```python
from build123d import *

# Parameters (mm, degrees)
BOSS_EXTRUDE1_DEPTH = 50.8
SKETCH2_R           = 8.636
SKETCH2_R_2         = 4.064
CUT_EXTRUDE1_DEPTH  = 50.8
CIRPATTERN1_COUNT   = 4


with BuildPart() as part:
    # Sketch1 → Boss-Extrude1 (new body)
    with BuildSketch(Plane.XY):
        with BuildLine():
            Line((-3.797752579, 127.26397791), (-3.797752579, 92.878939343))
            ThreePointArc((-3.797752579, 92.878939343), (0, 89.081186764), (3.797752579, 92.878939343))
            Line((3.797752579, 92.878939343), (3.797752579, 127.26397791))
            ThreePointArc((3.797752579, 127.26397791), (6.790630722, 127.103835386), (9.749331178, 126.62523659))
            ThreePointArc((9.749331178, 126.62523659), (30.88440355, 95.052420362), (66.541072029, 108.172481405))
            ThreePointArc((66.541072029, 108.172481405), (69.216024294, 106.82059547), (71.731442986, 105.190983859))
            Line((71.731442986, 105.190983859), (51.520424417, 77.372903306))
            ThreePointArc((51.520424417, 77.372903306), (52.360607836, 72.068193971), (57.665317172, 72.90837739))
            Line((57.665317172, 72.90837739), (77.876335741, 100.726457943))
            ThreePointArc((77.876335741, 100.726457943), (80.203495606, 98.837730286), (82.315821243, 96.711455232))
            ThreePointArc((82.315821243, 96.711455232), (80.856418217, 58.745626497), (117.415047369, 48.40151497))
            ThreePointArc((117.415047369, 48.40151497), (118.784510595, 45.735518782), (119.861665394, 42.938609284))
            Line((119.861665394, 42.938609284), (87.159550401, 32.313048015))
            ThreePointArc((87.159550401, 32.313048015), (84.721243151, 27.527600589), (89.506690576, 25.089293339))
            Line((89.506690576, 25.089293339), (122.208805569, 35.714854608))
            ThreePointArc((122.208805569, 35.714854608), (122.981351186, 32.818971587), (123.440465405, 29.857185076))
            ThreePointArc((123.440465405, 29.857185076), (99.944029333, 0), (123.440465405, -29.857185076))
            ThreePointArc((123.440465405, -29.857185076), (122.981351186, -32.818971587), (122.208805569, -35.714854608))
            Line((122.208805569, -35.714854608), (89.506690576, -25.089293339))
            ThreePointArc((89.506690576, -25.089293339), (84.721243151, -27.527600589), (87.159550401, -32.313048015))
            Line((87.159550401, -32.313048015), (119.861665394, -42.938609284))
            ThreePointArc((119.861665394, -42.938609284), (118.784510595, -45.735518782), (117.415047369, -48.40151497))
            ThreePointArc((117.415047369, -48.40151497), (80.856418217, -58.745626497), (82.315821243, -96.711455232))
            ThreePointArc((82.315821243, -96.711455232), (80.203495606, -98.837730286), (77.876335741, -100.726457943))
            Line((77.876335741, -100.726457943), (57.665317172, -72.90837739))
            ThreePointArc((57.665317172, -72.90837739), (52.360607836, -72.068193971), (51.520424417, -77.372903306))
            Line((51.520424417, -77.372903306), (71.731442986, -105.190983859))
            ThreePointArc((71.731442986, -105.190983859), (69.216024294, -106.82059547), (66.541072029, -108.172481405))
            ThreePointArc((66.541072029, -108.172481405), (30.88440355, -95.052420362), (9.749331178, -126.62523659))
            ThreePointArc((9.749331178, -126.62523659), (6.790630722, -127.103835386), (3.797752579, -127.26397791))
            Line((3.797752579, -127.26397791), (3.797752579, -92.878939343))
            ThreePointArc((3.797752579, -92.878939343), (0, -89.081186764), (-3.797752579, -92.878939343))
            Line((-3.797752579, -92.878939343), (-3.797752579, -127.26397791))
            ThreePointArc((-3.797752579, -127.26397791), (-6.790630722, -127.103835386), (-9.749331178, -126.62523659))
            ThreePointArc((-9.749331178, -126.62523659), (-30.88440355, -95.052420362), (-66.541072029, -108.172481405))
            ThreePointArc((-66.541072029, -108.172481405), (-69.216024294, -106.82059547), (-71.731442986, -105.190983859))
            Line((-71.731442986, -105.190983859), (-51.520424417, -77.372903306))
            ThreePointArc((-51.520424417, -77.372903306), (-52.360607836, -72.068193971), (-57.665317172, -72.90837739))
            Line((-57.665317172, -72.90837739), (-77.876335741, -100.726457943))
            ThreePointArc((-77.876335741, -100.726457943), (-80.203495606, -98.837730286), (-82.315821243, -96.711455232))
            ThreePointArc((-82.315821243, -96.711455232), (-80.856418217, -58.745626497), (-117.415047369, -48.40151497))
            ThreePointArc((-117.415047369, -48.40151497), (-118.784510595, -45.735518782), (-119.861665394, -42.938609284))
            Line((-119.861665394, -42.938609284), (-87.159550401, -32.313048015))
            ThreePointArc((-87.159550401, -32.313048015), (-84.721243151, -27.527600589), (-89.506690576, -25.089293339))
            Line((-89.506690576, -25.089293339), (-122.208805569, -35.714854608))
            ThreePointArc((-122.208805569, -35.714854608), (-122.981351186, -32.818971587), (-123.440465405, -29.857185076))
            ThreePointArc((-123.440465405, -29.857185076), (-99.944029333, 0), (-123.440465405, 29.857185076))
            ThreePointArc((-123.440465405, 29.857185076), (-122.981351186, 32.818971587), (-122.208805569, 35.714854608))
            Line((-122.208805569, 35.714854608), (-89.506690576, 25.089293339))
            ThreePointArc((-89.506690576, 25.089293339), (-84.721243151, 27.527600589), (-87.159550401, 32.313048015))
            Line((-87.159550401, 32.313048015), (-119.861665394, 42.938609284))
            ThreePointArc((-119.861665394, 42.938609284), (-118.784510595, 45.735518782), (-117.415047369, 48.40151497))
            ThreePointArc((-117.415047369, 48.40151497), (-80.856418217, 58.745626497), (-82.315821243, 96.711455232))
            ThreePointArc((-82.315821243, 96.711455232), (-80.203495606, 98.837730286), (-77.876335741, 100.726457943))
            Line((-77.876335741, 100.726457943), (-57.665317172, 72.90837739))
            ThreePointArc((-57.665317172, 72.90837739), (-52.360607836, 72.068193971), (-51.520424417, 77.372903306))
            Line((-51.520424417, 77.372903306), (-71.731442986, 105.190983859))
            ThreePointArc((-71.731442986, 105.190983859), (-69.216024294, 106.82059547), (-66.541072029, 108.172481405))
            ThreePointArc((-66.541072029, 108.172481405), (-30.88440355, 95.052420362), (-9.749331178, 126.62523659))
            ThreePointArc((-9.749331178, 126.62523659), (-6.790630722, 127.103835386), (-3.797752579, 127.26397791))
        make_face()
    extrude(amount=BOSS_EXTRUDE1_DEPTH)

    # Sketch2 → Cut-Extrude1 (cut)
    with BuildSketch(Plane(origin=(0, 0, 0), x_dir=(-1, 0, 0), z_dir=(0, 0, -1))):
        Circle(SKETCH2_R)
        with Locations((0, 26.162)):
            Circle(SKETCH2_R_2)
    cut_extrude1 = extrude(amount=-CUT_EXTRUDE1_DEPTH, mode=Mode.SUBTRACT)

    # CirPattern1: Cut-Extrude1 ×4 about axis
    cirpattern1_axis = Axis((0, 0, 0), (0, 0, 1))
    for i in range(1, CIRPATTERN1_COUNT):
        add(cut_extrude1.rotate(cirpattern1_axis, i * 360 / CIRPATTERN1_COUNT), mode=Mode.SUBTRACT)


solid = part.part
```
Design review of the part built by this model. Coordinates are the model's own, in mm. A direction names the side the tool comes from. Round coordinates to 2 decimals unless told otherwise and drop trailing zeros. Order: outer loops, then holes, each group sorted by start corner. A loop starts at its lowest first (then second) coordinate and runs counter-clockwise, first axis right, second up. Notation, with made-up numbers: (52, -21) - (109, -21) arc R24 ccw to (109, -2) - close; hole circle Ø7 at (-37, 41.5). An arc over 180 degrees is marked (long way). Return JSON: item names as keys, results as strings.
Q1. Wall thickness on L1, parallel to Y at x = 0, z = 22; L2, parallel to X at y = 0, z = 34; L3, parallel to X at y = -85.5, z = 23.5: over which ranges is each line inside the solid? List them lowest first. Write a range as [from, to].
Computed values:
{"L1": "y = [-89.08, -30.23], [-22.1, -8.64], [8.64, 22.1], [30.23, 89.08]", "L2": "x = [-99.94, -30.23], [-22.1, -8.64], [8.64, 22.1], [30.23, 99.94]", "L3": "x = [-76.25, -66.81], [-57.43, 57.43], [66.81, 76.25]"}
Q2. Consider section C-C on y = 111.5. Write out the cut boundary in (x, z).
Computed values:
{"outline": "(-12.44, 0) - (-3.8, 0) - (-3.8, 50.8) - (-12.44, 50.8) - close; (3.8, 0) - (12.44, 0) - (12.44, 50.8) - (3.8, 50.8) - close"}
Q3. The part is to be moulded in two halves that separate along X. For faces 1 (the cylindrical face through (122.973, 32.86, 25.044)), 2 (the flat face through (3.798, 110, 25)), 3 (the cylindrical face through (-6.83, 127.1, 25.04)), say which applies: pulls with the +X half, pulls with the -X half, needs draft (parallel to the pull), parting line crosses it, or undercut.
Computed values:
{"face 1": "pulls with the +X half", "face 2": "undercut", "face 3": "pulls with the -X half"}
Q4. Machinability: for faces 4 (the cylindrical face through (-99.95, -0.57, 25.04)), 5 (the flat face through (61.484, -91.087, 25.044)), which of the approach directions +Z, -Z, +X, -X, +Y, -Y give a long, thin tool a straight path to every point of the face, cutting with its end or side? Answer none if there is none.
Computed values:
{"face 4": "+Z, -Z, -X", "face 5": "+Z, -Z"}
Q5. Consider section D-D on z = 32. Give the number of separate pieces and of enclosed holes in the cut face, plus the area to 3 significant figures.
Computed values:
{"separate pieces": "1", "enclosed holes": "5", "area": "35,600 mm2"}
Q6. Consider section B-B on y = 0. Write out the cut boundary in (x, z).
Computed values:
{"outline": "(-99.94, 0) - (-30.23, 0) - (-30.23, 50.8) - (-99.94, 50.8) - close; (-22.1, 0) - (-8.64, 0) - (-8.64, 50.8) - (-22.1, 50.8) - close; (8.64, 0) - (22.1, 0) - (22.1, 50.8) - (8.64, 50.8) - close; (30.23, 0) - (99.94, 0) - (99.94, 50.8) - (30.23, 50.8) - close"}
Q7. For pin 1 Ø5 at (x, z) = (-83, 14) entering from -Y; pin 2 Ø1.5 at (x, z) = (-19.5, 13) entering from +Y; pin 3 Ø8 at (y, z) = (55, 17.5) entering from +X; pin 4 Ø9.5 at (x, y) = (26.162, 0) entering from -Z, all flat-tipped, find the tip position at first contact; note any pin that passes through.
Computed values:
{"pin 1": "stops at y = -98.57", "pin 2": "stops at y = 102.45", "pin 3": "stops at x = 89.04", "pin 4": "stops at z = 0"}
Q8. Consider section A-A on x = 0. Write out the cut boundary in (y, z), plus the area to 3 significant figures.
Computed values:
{"outline": "(-89.08, 0) - (-30.23, 0) - (-30.23, 50.8) - (-89.08, 50.8) - close; (-22.1, 0) - (-8.64, 0) - (-8.64, 50.8) - (-22.1, 50.8) - close; (8.64, 0) - (22.1, 0) - (22.1, 50.8) - (8.64, 50.8) - close; (30.23, 0) - (89.08, 0) - (89.08, 50.8) - (30.23, 50.8) - close", "area": "7,350 mm2"}
